Geometry check sheet. Reference: the model listing, model coordinates, mm. A direction names the side the tool comes from. Round coordinates to 2 decimals unless told otherwise and drop trailing zeros. Loops run counter-clockwise (first coordinate to the right, second up) from the corner with the lowest first, then second, coordinate; pieces in that order, holes last.
```python
from build123d import *

# Parameters (mm, degrees)
SKETCH1_W           = 10
SKETCH1_H           = 20
BOSS_EXTRUDE1_DEPTH = 20
SKETCH2_W           = 10
SKETCH2_H           = 17
CUT_EXTRUDE1_DEPTH  = 17
SKETCH3_R           = 2.5
CUT_EXTRUDE2_DEPTH  = 21
SKETCH4_W           = 10
SKETCH4_H           = 3
CUT_EXTRUDE3_DEPTH  = 4
SKETCH5_R           = 2
CUT_EXTRUDE4_DEPTH  = 4
FILLET1_R           = 1
SKETCH6_R           = 2.5
CUT_EXTRUDE5_DEPTH  = 4


with BuildPart() as part:
    # Sketch1 → Boss-Extrude1 (new body)
    with BuildSketch(Plane(origin=(0, 0, 0), x_dir=(1, 0, 0), z_dir=(0, 1, 0))):
        with Locations((5, 10)):
            Rectangle(SKETCH1_W, SKETCH1_H)
    extrude(amount=BOSS_EXTRUDE1_DEPTH)

    # Sketch2 → Cut-Extrude1 (cut)
    with BuildSketch(Plane(origin=(0, 20, 0), x_dir=(1, 0, 0), z_dir=(0, 1, 0))):
        with Locations((5, 11.5)):
            Rectangle(SKETCH2_W, SKETCH2_H)
    extrude(amount=-CUT_EXTRUDE1_DEPTH, mode=Mode.SUBTRACT)

    # Sketch3 → Cut-Extrude2 (cut, through all)
    with BuildSketch(Plane.XY):
        with Locations((5, 15)):
            Circle(SKETCH3_R)
    extrude(amount=-CUT_EXTRUDE2_DEPTH, mode=Mode.SUBTRACT)

    # Sketch4 → Cut-Extrude3 (cut, through all)
    with BuildSketch(Plane(origin=(0, 3, 0), x_dir=(1, 0, 0), z_dir=(0, 1, 0))):
        with Locations((5, 18.5)):
            Rectangle(SKETCH4_W, SKETCH4_H)
    extrude(amount=-CUT_EXTRUDE3_DEPTH, mode=Mode.SUBTRACT)

    # Sketch5 → Cut-Extrude4 (cut, through all)
    with BuildSketch(Plane(origin=(0, 3, 0), x_dir=(1, 0, 0), z_dir=(0, 1, 0))):
        with Locations((5, 6.5)):
            Circle(SKETCH5_R)
        with Locations((5, 13.5)):
            Circle(SKETCH5_R)
    extrude(amount=-CUT_EXTRUDE4_DEPTH, mode=Mode.SUBTRACT)

    # Fillet1
    fillet1_edges = [part.edges().sort_by_distance(p)[0] for p in [
        (10, 20, -1.5),
        (0, 20, -1.5),
        (0, 11.5, -3),
        (10, 3, -10),
        (5, 3, -3),
        (10, 11.5, -3),
        (5, 20, -3),
        (0, 3, -10),
        (0, 0, -8.5),
        (10, 0, -8.5),
        (5, 0, 0),
        (10, 10, 0),
        (0, 10, 0),
        (5, 20, 0),
    ]]
    fillet(fillet1_edges, radius=FILLET1_R)

    # Sketch6 → Cut-Extrude5 (cut, through all)
    with BuildSketch(Plane(origin=(0, 0, -3), x_dir=(-1, 0, 0), z_dir=(0, 0, -1))):
        with Locations((-4.5, 7)):
            Circle(SKETCH6_R)
    extrude(amount=-CUT_EXTRUDE5_DEPTH, mode=Mode.SUBTRACT)


solid = part.part
```
1) Scan lines: line 1 along Z through (x, y) = (5, 1.25); line 2 along X through (y, z) = (2.1, -6.5); line 3 along X through (y, z) = (9.25, -1.5). Record each from-to range of solid material in increasing order.
Report:
line 1: z = -17 to -15.5, -11.5 to -8.5, -4.5 to 0
line 2: x = 0.01 to 3, 7 to 9.99
line 3: x = 0 to 3.41, 5.59 to 10
2) Sectioned sample at C-C, the plane z = -1.5. Record the cut outline in (x, y), then the cut area to 3 significant figures.
Report:
outline: (0, 1) arc R1 ccw to (1, 0) - (9, 0) arc R1 ccw to (10, 1) - (10, 19) arc R1 ccw to (9, 20) - (1, 20) arc R1 ccw to (0, 19) - close; hole circle Ø5 at (4.5, 7); hole circle Ø5 at (5, 15)
area: 160 mm2
3) Gauge pin test, flat ends, axial feed: pin 1 (1.5 mm diameter, centred on x = 6.5, z = -10, fed in from +Y); pin 2 (1.5 mm diameter, centred on y = 7, z = -3, fed in from +X); pin 3 (2.5 mm diameter, centred on x = 3.5, y = 12, fed in from -Z); pin 4 (4.5 mm diameter, centred on x = 5, z = -6.5, fed in from -Y). Record the tip position at first contact, or that the pin passes through.
Report:
pin 1: stops at y = 3
pin 2: stops at x = 9.97
pin 3: stops at z = -3
pin 4: stops at y = 0
4) Sectioned sample at B-B, the plane z = -6.5. Record the cut outline in (x, y), then the cut area to 3 significant figures.
Report:
outline: (0, 1) arc R1 ccw to (1, 0) - (3, 0) - (3, 3) - (1, 3) arc R1 ccw to (0, 2) - close; (7, 0) - (9, 0) arc R1 ccw to (10, 1) - (10, 2) arc R1 ccw to (9, 3) - (7, 3) - close
area: 17.1 mm2
5) Sectioned sample at D-D, the plane x = 5. Record the cut outline in (y, z), then the cut area to 3 significant figures.
Report:
outline: (0, -17) - (3, -17) - (3, -15.5) - (0, -15.5) - close; (0, -11.5) - (3, -11.5) - (3, -8.5) - (0, -8.5) - close; (0, -4.5) - (3, -4.5) - (3, -4) arc R1 cw to (4, -3) - (4.55, -3) - (4.55, 0) - (1, 0) arc R1 ccw to (0, -1) - close; (9.45, -3) - (12.5, -3) - (12.5, 0) - (9.45, 0) - close; (17.5, -3) - (19, -3) arc R1 ccw to (20, -2) - (20, -1) arc R1 ccw to (19, 0) - (17.5, 0) - close
area: 47.9 mm2
6) Mould release check, pull along Y, two halves, no side actions. Record for faces 3 (the face through (3, 5, -2)), 4 (the face through (5, 3, -11)), 5 (the face through (9.699, 10.126, -0.285)), 6 (the face through (9.699, 0.285, -9.112)): +Y half, -Y half, draft (parallel to the pull), parting line (faces both ways), or undercut.
Report:
face 3: undercut
face 4: +Y half
face 5: draft
face 6: -Y half
7) Access from +Z, -Z, +X, -X, +Y, -Y to the whole of each face (thin tool, end or side, straight path). Record for faces 1 (the face through (9.699, 2.715, -10.591)), 2 (the face through (5.056, 0.285, -0.301)).
Report:
face 1: -Z, +X, +Y
face 2: +Z, +X, -X, -Y
8) Sectioned sample at A-A, the plane y = 15. Record the cut outline in (x, z).
Report:
outline: (0, -2) arc R1 ccw to (1, -3) - (2.5, -3) - (2.5, 0) - (1, 0) arc R1 ccw to (0, -1) - close; (7.5, -3) - (9, -3) arc R1 ccw to (10, -2) - (10, -1) arc R1 ccw to (9, 0) - (7.5, 0) - close
